```python
from build123d import *

# Parameters (mm, degrees)
SKETCH_1_R      = 10
SKETCH_1_R_2    = 4
EXTRUDE_1_DEPTH = 10
CHAMFER_1_SIZE  = 0.3
EXTRUDE_2_DEPTH = 9


with BuildPart() as part:
    # 스케치1 → 보스-돌출1 (new body)
    with BuildSketch(Plane.XY):
        Circle(SKETCH_1_R)
        Circle(SKETCH_1_R_2, mode=Mode.SUBTRACT)
    extrude(amount=EXTRUDE_1_DEPTH)

    # 모따기1
    chamfer_1_edges = [part.edges().sort_by_distance(p)[0] for p in [
        (-10, 0, 0),
        (-4, 0, 0),
    ]]
    chamfer(chamfer_1_edges, length=CHAMFER_1_SIZE)

    # 스케치2 → 보스-돌출2 (add)
    with BuildSketch(Plane.XY.offset(10)):
        with BuildLine():
            ThreePointArc((-3.5, 9.367496998), (-7.071067812, 7.071067812), (-9.367496998, 3.5))
            Line((-9.367496998, 3.5), (-3.5, 3.5))
            Line((-3.5, 3.5), (-3.5, 9.367496998))
        make_face()
        with BuildLine():
            Line((9.367496998, -3.5), (3.5, -3.5))
            Line((3.5, -3.5), (3.5, -9.367496998))
            ThreePointArc((3.5, -9.367496998), (7.071067812, -7.071067812), (9.367496998, -3.5))
        make_face()
    extrude(amount=EXTRUDE_2_DEPTH)

    # 스케치3 → 컷-회전1 (revolve, cut)
    with BuildSketch(Plane(origin=(0, 0, 0), x_dir=(1, 0, 0), z_dir=(0, 1, 0)), mode=Mode.PRIVATE) as cut_revolve_1_sk:
        Polygon((9.133974596, -10), (10, -10.5), (10, -9.5), align=None)
    revolve(cut_revolve_1_sk.sketch.rotate(Axis((0, 0, 0), (0, 0, 1)), 180), axis=Axis((0, 0, 0), (0, 0, 1)), mode=Mode.SUBTRACT)


solid = part.part
```
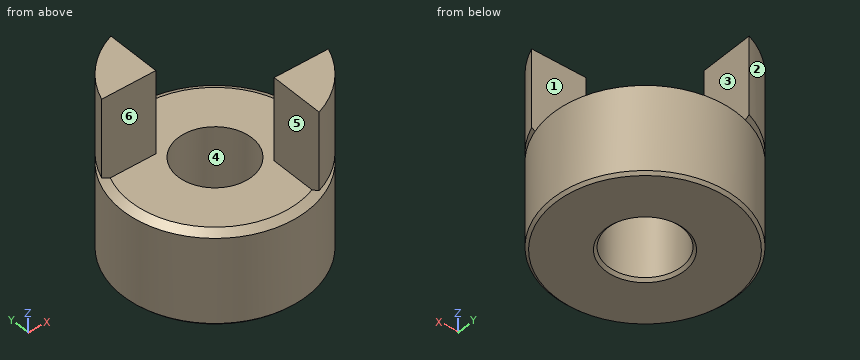
The listing builds one solid part. Answer for the finished solid, in the listing's coordinates (mm). Face numbers are marked on the shaded views. A direction names the side the tool comes from. Coordinates: 2 decimals unless noted, no trailing zeros. Write each loop counter-clockwise with the first axis right and the second up, starting at its lowest first coordinate (ties: lowest second). Pieces come first, ordered by that corner, then holes. Notation, with made-up numbers: M 84,83.25 L 88,83.25 A20 cw 88,111.25 Z; hole C 49,-33.5 d1. An arc over 180 degrees is marked long. Use a Markdown table: item, result. Add a question column.
1. Section A-A (y = 0) is taken. Give the vertices of the cut face in (x, z).
2. Section D-D (z = 3) is taken. Give the vertices of the cut face in (x, y), plus the area to 3 significant figures.
3. Section C-C (z = 17.25) is taken. Give the vertices of the cut face in (x, y), plus the area to 3 significant figures.
4. For a pull along X with two mould halves and no side action, classify the marked faces 4, 5 and 6 as +X half, -X half, draft (parallel to the pull), parting line (faces both ways), or undercut.
5. Straight lines are drawn through the part: line 1 along Y through (x, z) = (0, 4); line 2 along Z through (x, y) = (5.75, -0.75); line 3 along X through (y, z) = (-2.75, 8.5). For each, find the intervals that lie inside material, in ascending order. Write a range as [from, to].
6. Given P1, Ø2, axis at y = 3.5, z = 12.5, coming from the +X side; P2, Ø5, axis at y = -5, z = 11.5, coming from the -X side; P3, Ø6.5, axis at x = -7, z = 15, coming from the -Y side, each flat-ended and moving along its own axis, determine where each tip first touches the part or whether it passes through.
7. Which of the six approach directions +Z, -Z, +X, -X, +Y, -Y give full straight-line access (tool end or side, diameter ignored) to the marked faces 1, 2 and 3?
Data:
| question | item | result |
|---|---|---|
| 1 | outline | M -10,0.3 L -9.7,0 L -4.3,0 L -4,0.3 L -4,10 L -9.13,10 L -10,9.5 Z; M 4,0.3 L 4.3,0 L 9.7,0 L 10,0.3 L 10,9.5 L 9.13,10 L 4,10 Z |
| 2 | outline | C 0,0 d20; hole C 0,0 d8 |
| 2 | area | 264 mm2 |
| 3 | outline | M -9.37,3.5 L -3.5,3.5 L -3.5,9.37 A10 ccw Z; M 3.5,-9.37 A10 ccw 9.37,-3.5 L 3.5,-3.5 Z |
| 3 | area | 44.5 mm2 |
| 4 | face 4 | undercut |
| 4 | face 5 | -X half |
| 4 | face 6 | draft |
| 5 | line 1 | y = [-10, -4], [4, 10] |
| 5 | line 2 | z = [0, 10] |
| 5 | line 3 | x = [-9.61, -2.9], [2.9, 9.61] |
| 6 | P1 | stops at x = -3.5 |
| 6 | P2 | stops at x = -9.37 |
| 6 | P3 | stops at y = 3.5 |
| 7 | face 1 | +Z, +X, -X, +Y |
| 7 | face 2 | +Z, -Z, -X, +Y |
| 7 | face 3 | +Z, +X, +Y, -Y |
